Could you check a few things on this drawing? It's one solid part, dimensions in mm from its lowest x, y, z. A direction names the side the tool comes from. Coordinates: 2 decimals unless noted, no trailing zeros. Write each loop counter-clockwise with the first axis right and the second up, starting at its lowest first coordinate (ties: lowest second). Pieces come first, ordered by that corner, then holes. Notation, with made-up numbers: (-19, 43) - (6, 43) arc R33 cw to (6, 73) - close; hole circle Ø5 at (2, 62.5). An arc over 180 degrees is marked (long way). Use one line per item in the form item = value. Start each with the question number.
(1) If I drill on probe 1 along X at (y, z) = (47.5, 2); probe 2 along Z at (x, y) = (63, 6); probe 3 along Z at (x, y) = (98, 3.5), over which ranges is the centre line in solid material (lowest first)? Write a range as from..to.
(2) If we section it at B-B on x = 93: Please give me the cut outline in (y, z).
(3) On a 3-axis mill with a long thin cutter (end or side, diameter ignored), from which of +Z, -Z, +X, -X, +Y, -Y can I reach the whole of each face in a straight line? I mean the marked faces 1 and 2. Say none if no direction works.
(4) Thinking about a two-plate mould opening in X: for the marked faces 3, 4 and 5, which applies, pulls with the +X half, pulls with the -X half, needs draft (parallel to the pull), parting line crosses it, or undercut?
(5) If we section it at C-C on y = 6: Please give me the cut outline in (x, z), then the cut area to 3 significant figures.
(6) For pin 1 Ø4 at (x, z) = (91.5, 13) entering from -Y; pin 2 Ø7.5 at (x, z) = (53.5, 5) entering from +Y, each with a flat end and sliding along its axis, tell me the tip position at first contact or that it passes through.
(7) If we section it at A-A on y = 46.5: Please give me the cut outline in (x, z), then the cut area to 3 significant figures.
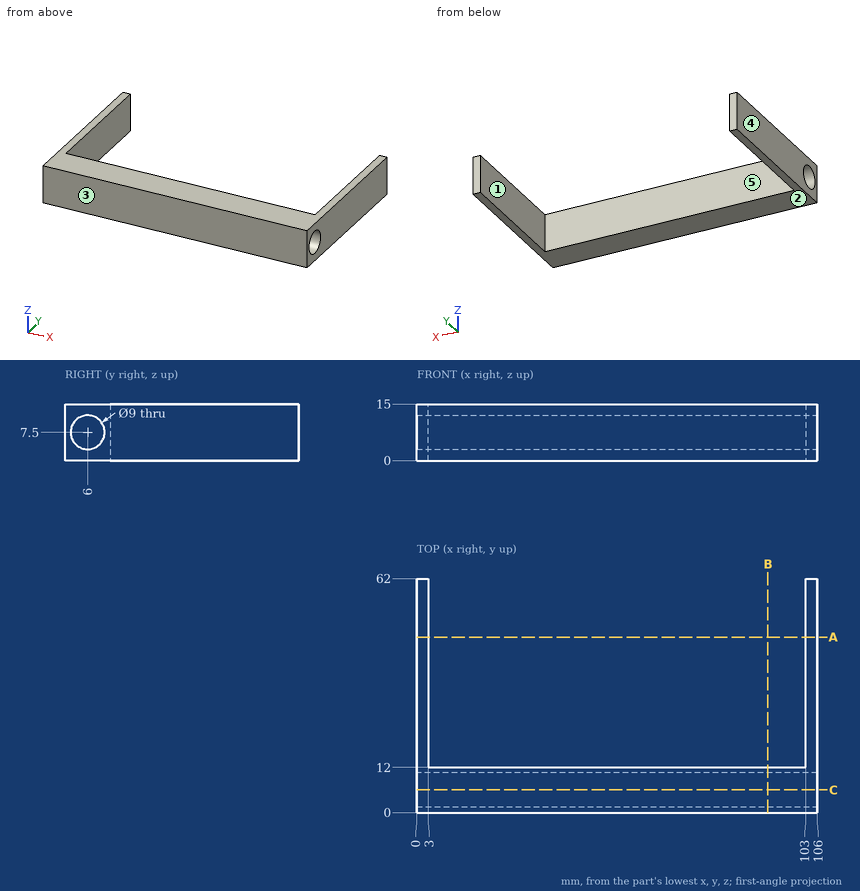
Reported:
q1.probe_1 = 0..3, 103..106
q1.probe_2 = 0..3, 12..15
q1.probe_3 = 0..3.76, 11.24..15
q2.outline = (0, 0) - (12, 0) - (12, 15) - (0, 15) - close; hole circle Ø9 at (6, 7.5)
q3.face_1 = +Z, -Z, +Y
q3.face_2 = -Z, +X, -X, +Y, -Y
q4.face_3 = needs draft
q4.face_4 = pulls with the -X half
q4.face_5 = undercut
q5.outline = (0, 0) - (106, 0) - (106, 3) - (0, 3) - close; (0, 12) - (106, 12) - (106, 15) - (0, 15) - close
q5.area = 636 mm2
q6.pin_1 = 0
q6.pin_2 = 12
q7.outline = (0, 0) - (3, 0) - (3, 15) - (0, 15) - close; (103, 0) - (106, 0) - (106, 15) - (103, 15) - close
q7.area = 90.0 mm2
